Print and shaded views of the part. All mm, measured from the part's lowest x, y and z. Give positions to 0.01 mm unless a question says otherwise; leave off trailing zeros. Loops run counter-clockwise (first coordinate to the right, second up) from the corner with the lowest first, then second, coordinate; pieces in that order, holes last.
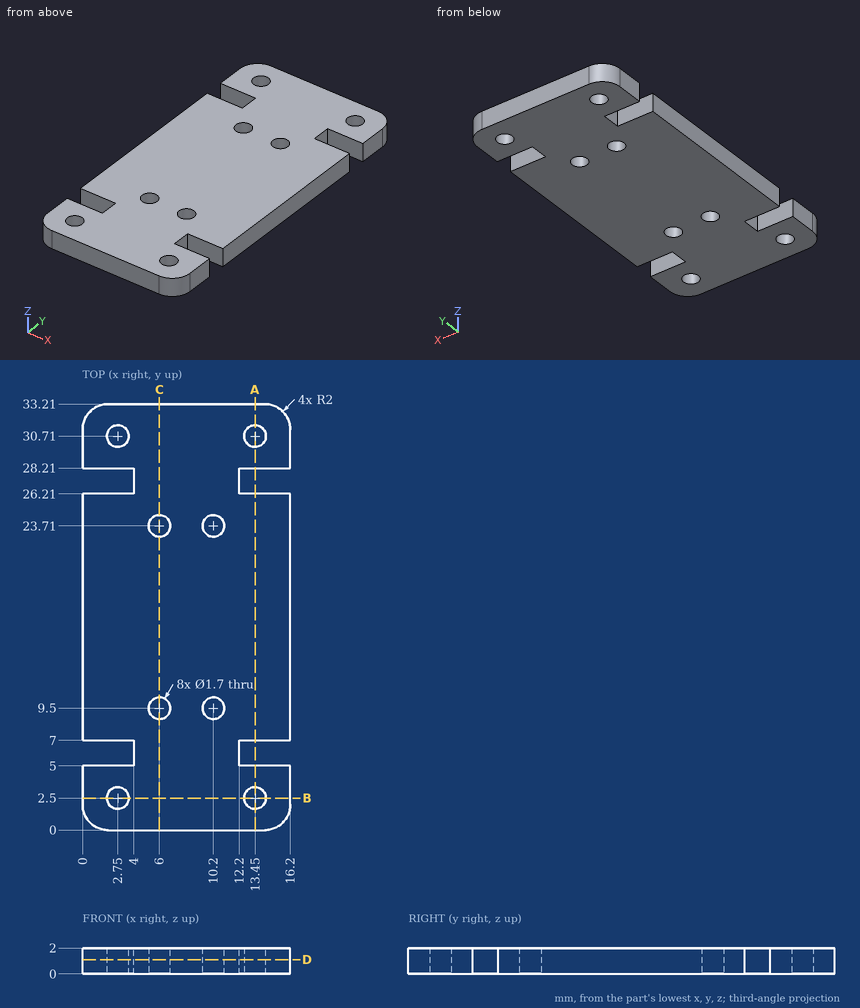
1. Drop flat-ended pins along their axis: pin 1 (1.4 mm diameter, centred on x = 2.75, y = 2.5, fed in from -Z); pin 2 (1 mm diameter, centred on y = 6, z = 1, fed in from -X); pin 3 (0.6 mm diameter, centred on x = 15, z = 0.5, fed in from -Y). Give the stop position or say it passes through.
Responses:
pin 1: passes through
pin 2: stops at x = 4
pin 3: stops at y = 0.06
2. Probe line 1 along Y through (x, z) = (10.2, 0.75); line 2 along X through (y, z) = (23.71, 1.25); line 3 along Y through (x, z) = (13.45, 0.7). List the from-to ranges inside material, lowest first.
Responses:
line 1: y = 0 to 8.65, 10.35 to 22.86, 24.56 to 33.21
line 2: x = 0 to 5.15, 6.85 to 9.35, 11.05 to 16.2
line 3: y = 0 to 1.65, 3.35 to 5, 7 to 26.21, 28.21 to 29.86, 31.56 to 33.21
3. Saw through at D-D, the plane z = 1.1. Count the separate pieces of the cut face and the enclosed holes in it, and give its area (3 significant figures).
Responses:
separate pieces: 1
enclosed holes: 8
area: 484 mm2
4. Saw through at A-A, the plane x = 13.45. List the corners of the cut face in (y, z).
Responses:
outline: (0, 0) - (1.65, 0) - (1.65, 2) - (0, 2) - close; (3.35, 0) - (5, 0) - (5, 2) - (3.35, 2) - close; (7, 0) - (26.21, 0) - (26.21, 2) - (7, 2) - close; (28.21, 0) - (29.86, 0) - (29.86, 2) - (28.21, 2) - close; (31.56, 0) - (33.21, 0) - (33.21, 2) - (31.56, 2) - close
5. Saw through at B-B, the plane y = 2.5. List the corners of the cut face in (x, z).
Responses:
outline: (0, 0) - (1.9, 0) - (1.9, 2) - (0, 2) - close; (3.6, 0) - (12.6, 0) - (12.6, 2) - (3.6, 2) - close; (14.3, 0) - (16.2, 0) - (16.2, 2) - (14.3, 2) - close
6. Saw through at C-C, the plane x = 6. List the corners of the cut face in (y, z), and give its area (3 significant figures).
Responses:
outline: (0, 0) - (8.65, 0) - (8.65, 2) - (0, 2) - close; (10.35, 0) - (22.86, 0) - (22.86, 2) - (10.35, 2) - close; (24.56, 0) - (33.21, 0) - (33.21, 2) - (24.56, 2) - close
area: 59.6 mm2
